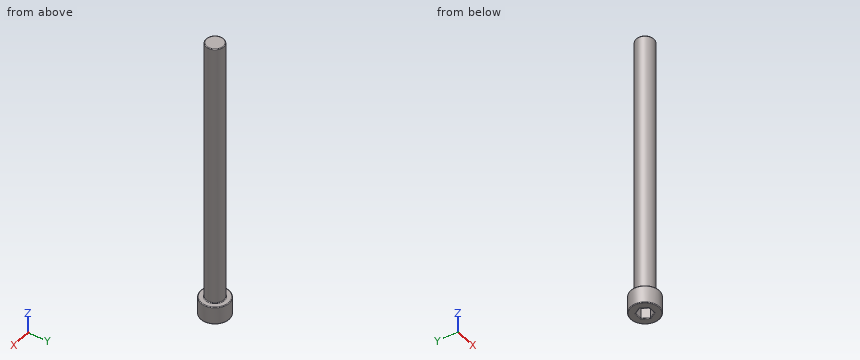
```python
from build123d import *

# Parameters (mm, degrees)
SKETCH_1_R          = 4
EXTRUDE_1_DEPTH     = 120
SKETCH_3_R          = 6.45
EXTRUDE_2_DEPTH     = 8
CUT_EXTRUDE_1_DEPTH = 5
FILLET_1_R          = 0.3


with BuildPart() as part:
    # Эскиз1 → Бобышка-Вытянуть1 (new body)
    with BuildSketch(Plane.XY):
        Circle(SKETCH_1_R)
    extrude(amount=EXTRUDE_1_DEPTH)

    # Эскиз3 → Бобышка-Вытянуть2 (add)
    with BuildSketch(Plane(origin=(0, 0, 0), x_dir=(-1, 0, 0), z_dir=(0, 0, -1))):
        Circle(SKETCH_3_R)
    extrude(amount=EXTRUDE_2_DEPTH)

    # Эскиз4 → Вырез-Вытянуть1 (cut)
    with BuildSketch(Plane(origin=(0, 0, -8), x_dir=(-1, 0, 0), z_dir=(0, 0, -1))):
        Polygon((-3.464101615, 0), (-1.732050808, -3), (1.732050808, -3), (3.464101615, 0), (1.732050808, 3), (-1.732050808, 3), align=None)
    extrude(amount=-CUT_EXTRUDE_1_DEPTH, mode=Mode.SUBTRACT)

    # Скругление1
    fillet_1_edges = [part.edges().sort_by_distance(p)[0] for p in [
        (2.598076211, 1.5, -3),
        (0, 3, -3),
        (-2.598076211, 1.5, -3),
        (-2.598076211, -1.5, -3),
        (0, -3, -3),
        (2.598076211, -1.5, -3),
        (2.598076211, 1.5, -8),
        (2.598076211, -1.5, -8),
        (0, -3, -8),
        (-2.598076211, -1.5, -8),
        (-2.598076211, 1.5, -8),
        (0, 3, -8),
        (-4, 0, 120),
        (-4, 0, 0),
        (6.45, 0, 0),
        (6.45, 0, -8),
    ]]
    fillet(fillet_1_edges, radius=FILLET_1_R)


solid = part.part
```
Work out the finished part from the listing and answer in its coordinate system (mm). Give positions to 0.01 mm unless a question says otherwise; leave off trailing zeros. Write each loop counter-clockwise with the first axis right and the second up, starting at its lowest first coordinate (ties: lowest second). Pieces come first, ordered by that corner, then holes. Notation, with made-up numbers: (83, -11.5) -> (133, -11.5) arc R19 cw to (133, -0.5) -> close; hole circle Ø5 at (5.25, 76). An arc over 180 degrees is marked (long way). Write item = value, one per line.
Q1. Flat-ended cylindrical pins translate along their axes: pin 1 Ø3 at (y, z) = (-3.5, 34.5) entering from -X; pin 2 Ø2.5 at (x, y) = (-1, -1.5) entering from -Z; pin 3 Ø3 at (y, z) = (-5, 7) entering from +X. Find the tip coordinate at first contact, or state that the pin passes through.
Computed values:
pin_1 = -3.46
pin_2 = -3.05
pin_3 = 1.94
Q2. Section B-B on z = 88 is taken. Determine the outline of the cut face in (x, y).
Computed values:
outline = circle Ø8 at (0, 0)
Q3. Section A-A on x = 0 is taken. Determine the outline of the cut face in (y, z), and give its area (3 significant figures).
Computed values:
outline = (-6.45, -7.7) arc R0.3 ccw to (-6.15, -8) -> (-3.3, -8) arc R0.3 ccw to (-3, -7.7) -> (-3, -3.3) arc R0.3 cw to (-2.7, -3) -> (2.7, -3) arc R0.3 cw to (3, -3.3) -> (3, -7.7) arc R0.3 ccw to (3.3, -8) -> (6.15, -8) arc R0.3 ccw to (6.45, -7.7) -> (6.45, -0.3) arc R0.3 ccw to (6.15, 0) -> (4.3, 0) arc R0.3 cw to (4, 0.3) -> (4, 119.7) arc R0.3 ccw to (3.7, 120) -> (-3.7, 120) arc R0.3 ccw to (-4, 119.7) -> (-4, 0.3) arc R0.3 cw to (-4.3, 0) -> (-6.15, 0) arc R0.3 ccw to (-6.45, -0.3) -> close
area = 1,030 mm^2
Q4. Consider line 1 along Z through (x, y) = (5.75, 0); line 2 along Z through (x, y) = (1.5, 0.5); line 3 along Y through (x, z) = (2.5, 6.5). Determine where each line is inside the solid, lowest interval first.
Computed values:
line_1 = -8 to 0
line_2 = -3 to 120
line_3 = -3.12 to 3.12
